Input: dimensioned drawing with shaded views. Units: mm. Origin: part minimum x, y, z. A direction names the side the tool comes from. Round coordinates to 2 decimals unless told otherwise and drop trailing zeros. Loops run counter-clockwise (first coordinate to the right, second up) from the corner with the lowest first, then second, coordinate; pieces in that order, holes last.
1) Section A-A, the plane x = 8.5. Return loops of the section in (y, z).
2) Section B-B, the plane z = 13. Return loops of the section in (x, y), and give its area (3 significant figures).
3) First-contact query: pin 1 (12 mm diameter, centred on x = 6.5, z = 15.5, fed in from +Y); pin 2 (4 mm diameter, centred on y = 4, z = 4, fed in from +X); pin 3 (3 mm diameter, centred on x = 8, z = 8, fed in from +Y); pin 4 (3 mm diameter, centred on x = 5.5, z = 19.5, fed in from -Y). Flat tips, straight axial feed; report the tip coordinate or a pass-through.
4) Access query for the marked faces 1, 2 and 3. Directions: +Z, -Z, +X, -X, +Y, -Y. A direction counts if a zero-diameter tool reaches every point of the face in a straight line with its end or side. Return the directions, or none.
5) Section C-C, the plane y = 6. Return loops of the section in (x, z), and give its area (3 significant figures).
6) Draft query along Y for the marked faces 4, 5 and 6. Return one class per face: pulls with the +Y half, pulls with the -Y half, needs draft (parallel to the pull), parting line crosses it, or undercut.
7) Ray query, line 1 along Z through (x, y) = (14, 4); line 2 along Y through (x, z) = (17.75, 4); line 3 along Z through (x, y) = (13, 4). Return the intervals inside material, ascending.
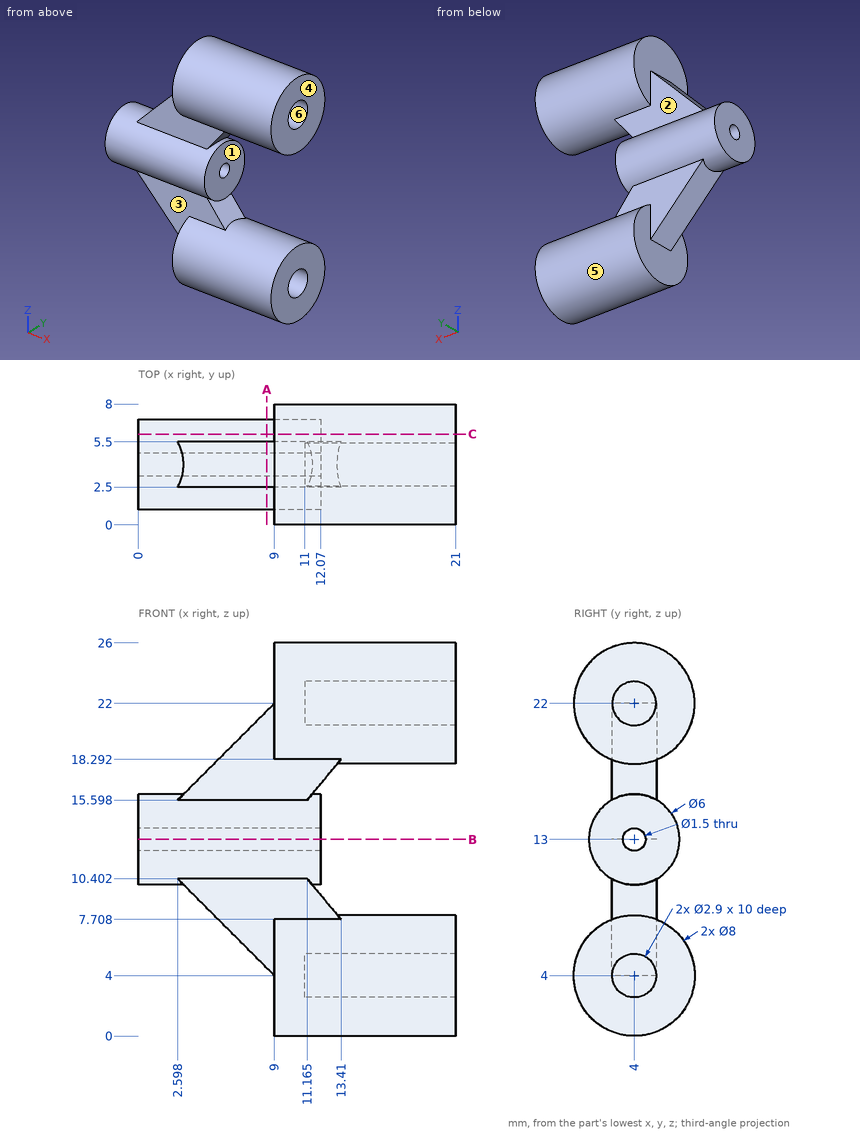
Final values:
1. outline: (2.5, 4.5) - (5.5, 4.5) - (5.5, 10.4) arc R3 ccw to (5.5, 15.6) - (5.5, 21.5) - (2.5, 21.5) - (2.5, 15.6) arc R3 ccw to (2.5, 10.4) - close; hole circle Ø1.5 at (4, 13)
2. outline: (0, 1) - (12.07, 1) - (12.07, 3.25) - (0, 3.25) - close; (0, 4.75) - (12.07, 4.75) - (12.07, 7) - (0, 7) - close
2. area: 54.3 mm2
3. pin 1: stops at y = 7.86
3. pin 2: stops at x = 21
3. pin 3: stops at y = 6.77
3. pin 4: stops at y = 2.5
4. face 1: +X, +Y, -Y
4. face 2: -X, +Y
4. face 3: -X, -Y
5. outline: (0, 10.76) - (12.07, 10.76) - (12.07, 15.24) - (0, 15.24) - close; (9, 0.54) - (21, 0.54) - (21, 7.46) - (9, 7.46) - close; (9, 18.54) - (21, 18.54) - (21, 25.46) - (9, 25.46) - close
5. area: 220 mm2
6. face 4: needs draft
6. face 5: parting line crosses it
6. face 6: undercut
7. line 1: z = 0 to 2.55, 5.45 to 8, 18 to 20.55, 23.45 to 26
7. line 2: y = 0 to 2.55, 5.45 to 8
7. line 3: z = 0 to 2.55, 5.45 to 8.2, 17.8 to 20.55, 23.45 to 26
